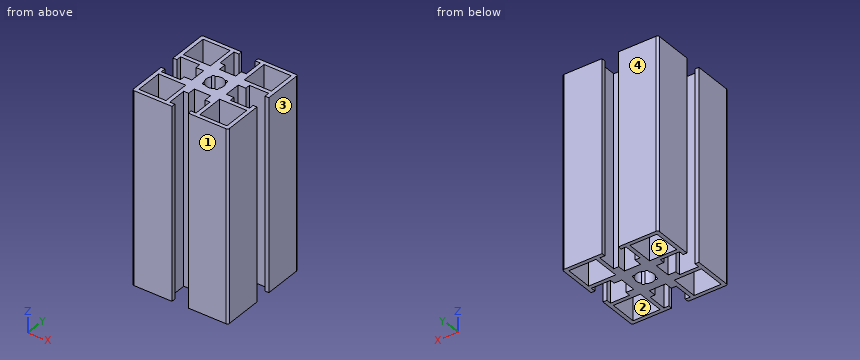
from build123d import *

# Parameters (mm, degrees)
SKETCH_1_W      = 14.15
SKETCH_1_H      = 14.15
EXTRUDE_1_DEPTH = 100


with BuildPart() as part:
    # 草图1 → 凸台-拉伸1 (new body)
    with BuildSketch(Plane.XY):
        with BuildLine():
            Line((-25, 24), (-25, 4.25))
            Line((-25, 4.25), (-23, 4.25))
            Line((-23, 4.25), (-23, 6.85))
            Line((-23, 6.85), (-13, 6.85))
            Line((-13, 6.85), (-13, 4.25))
            Line((-13, 4.25), (-9, 4.25))
            Line((-9, 4.25), (-9, -4.25))
            Line((-9, -4.25), (-13, -4.25))
            Line((-13, -4.25), (-13, -6.85))
            Line((-13, -6.85), (-23, -6.85))
            Line((-23, -6.85), (-23, -4.25))
            Line((-23, -4.25), (-25, -4.25))
            Line((-25, -4.25), (-25, -24))
            ThreePointArc((-25, -24), (-24.707106781, -24.707106781), (-24, -25))
            Line((-24, -25), (-4.25, -25))
            Line((-4.25, -25), (-4.25, -23))
            Line((-4.25, -23), (-6.85, -23))
            Line((-6.85, -23), (-6.85, -13))
            Line((-6.85, -13), (-4.25, -13))
            Line((-4.25, -13), (-4.25, -9))
            Line((-4.25, -9), (4.25, -9))
            Line((4.25, -9), (4.25, -13))
            Line((4.25, -13), (6.85, -13))
            Line((6.85, -13), (6.85, -23))
            Line((6.85, -23), (4.25, -23))
            Line((4.25, -23), (4.25, -25))
            Line((4.25, -25), (24, -25))
            ThreePointArc((24, -25), (24.707106781, -24.707106781), (25, -24))
            Line((25, -24), (25, -4.25))
            Line((25, -4.25), (23, -4.25))
            Line((23, -4.25), (23, -6.85))
            Line((23, -6.85), (13, -6.85))
            Line((13, -6.85), (13, -4.25))
            Line((13, -4.25), (9, -4.25))
            Line((9, -4.25), (9, 4.25))
            Line((9, 4.25), (13, 4.25))
            Line((13, 4.25), (13, 6.85))
            Line((13, 6.85), (23, 6.85))
            Line((23, 6.85), (23, 4.25))
            Line((23, 4.25), (25, 4.25))
            Line((25, 4.25), (25, 24))
            ThreePointArc((25, 24), (24.707106781, 24.707106781), (24, 25))
            Line((24, 25), (4.25, 25))
            Line((4.25, 25), (4.25, 23))
            Line((4.25, 23), (6.85, 23))
            Line((6.85, 23), (6.85, 13))
            Line((6.85, 13), (4.25, 13))
            Line((4.25, 13), (4.25, 9))
            Line((4.25, 9), (-4.25, 9))
            Line((-4.25, 9), (-4.25, 13))
            Line((-4.25, 13), (-6.85, 13))
            Line((-6.85, 13), (-6.85, 23))
            Line((-6.85, 23), (-4.25, 23))
            Line((-4.25, 23), (-4.25, 25))
            Line((-4.25, 25), (-24, 25))
            ThreePointArc((-24, 25), (-24.707106781, 24.707106781), (-25, 24))
        make_face()
        with Locations((15.925, 15.925)):
            Rectangle(SKETCH_1_W, SKETCH_1_H, mode=Mode.SUBTRACT)
        with Locations((15.925, -15.925)):
            Rectangle(SKETCH_1_W, SKETCH_1_H, mode=Mode.SUBTRACT)
        with Locations((-15.925, -15.925)):
            Rectangle(SKETCH_1_W, SKETCH_1_H, mode=Mode.SUBTRACT)
        with Locations((-15.925, 15.925)):
            Rectangle(SKETCH_1_W, SKETCH_1_H, mode=Mode.SUBTRACT)
        with BuildLine():
            ThreePointArc((-3.749249273, 2.665169767), (-4.599959429, -0.019319679), (-3.726730147, -2.696568636))
            ThreePointArc((-3.726730147, -2.696568636), (-3.767099489, -3.798876339), (-2.665169767, -3.749249273))
            ThreePointArc((-2.665169767, -3.749249273), (0.019319679, -4.599959429), (2.696568636, -3.726730147))
            ThreePointArc((2.696568636, -3.726730147), (3.798876339, -3.767099489), (3.749249273, -2.665169767))
            ThreePointArc((3.749249273, -2.665169767), (4.599959429, 0.019319679), (3.726730147, 2.696568636))
            ThreePointArc((3.726730147, 2.696568636), (3.767099489, 3.798876339), (2.665169767, 3.749249273))
            ThreePointArc((2.665169767, 3.749249273), (-0.019319679, 4.599959429), (-2.696568636, 3.726730147))
            ThreePointArc((-2.696568636, 3.726730147), (-3.798876339, 3.767099489), (-3.749249273, 2.665169767))
        make_face(mode=Mode.SUBTRACT)
    extrude(amount=EXTRUDE_1_DEPTH)


solid = part.part
Geometry: final body of the model. Coordinates: model frame, mm. Face numbers are marked on the shaded views. A direction names the side the tool comes from. Round coordinates to 2 decimals unless told otherwise and drop trailing zeros. Order: outer loops, then holes, each group sorted by start corner. A loop starts at its lowest first (then second) coordinate and runs counter-clockwise, first axis right, second up.
Q1. Section A-A, the plane x = -14.5. Output: boundary loops of the cut face in (y, z), and give its area (3 significant figures).
Result sheet:
outline: (-25, 0) - (-23, 0) - (-23, 100) - (-25, 100) - close; (-8.85, 0) - (-6.85, 0) - (-6.85, 100) - (-8.85, 100) - close; (6.85, 0) - (8.85, 0) - (8.85, 100) - (6.85, 100) - close; (23, 0) - (25, 0) - (25, 100) - (23, 100) - close
area: 800 mm2
Q2. Mould query, pull axis X, two halves, no side actions, for the marked faces 1, 2 and 3. Classes: released by +X, released by -X, zero draft, split by the parting line, or undercut.
Result sheet:
face 1: zero draft
face 2: undercut
face 3: released by +X
Q3. Pin query (flat end, axial travel): pin 1 (3 mm diameter, centred on x = -18, y = -3.5, fed in from -Z). Return the tip coordinate at first contact, or that it passes through.
Result sheet:
pin 1: passes through
Q4. Access query for the marked faces 4 and 5. Directions: +Z, -Z, +X, -X, +Y, -Y. A direction counts if a zero-diameter tool reaches every point of the face in a straight line with its end or side. Return the directions, or none.
Result sheet:
face 4: +Z, -Z, +X, -X, +Y
face 5: +Z, -Z
Q5. Material intervals for probe 1 along Y at (x, z) = (-12, 15); probe 2 along X at (y, z) = (-6.5, 71), sorted ascending.
Result sheet:
probe 1: y = -25 to -23, -8.85 to -4.25, 4.25 to 8.85, 23 to 25
probe 2: x = -25 to -23, -13 to 13, 23 to 25
Q6. Section B-B, the plane z = 15. Give the number of separate pieces and of enclosed holes in the cut face, and give its area (3 significant figures).
Result sheet:
separate pieces: 1
enclosed holes: 5
area: 876 mm2
